Part print with two shaded views. Sizes in mm from the minimum x, y, z corner. Give positions to 0.01 mm unless a question says otherwise; leave off trailing zeros. Loops run counter-clockwise (first coordinate to the right, second up) from the corner with the lowest first, then second, coordinate; pieces in that order, holes last. Notation, with made-up numbers: (-34, -24.75) -> (3, -24.75) arc R16 cw to (3, -14.75) -> close; hole circle Ø9 at (36, 46). An arc over 180 degrees is marked (long way). One line per question, with ' | ' between items.
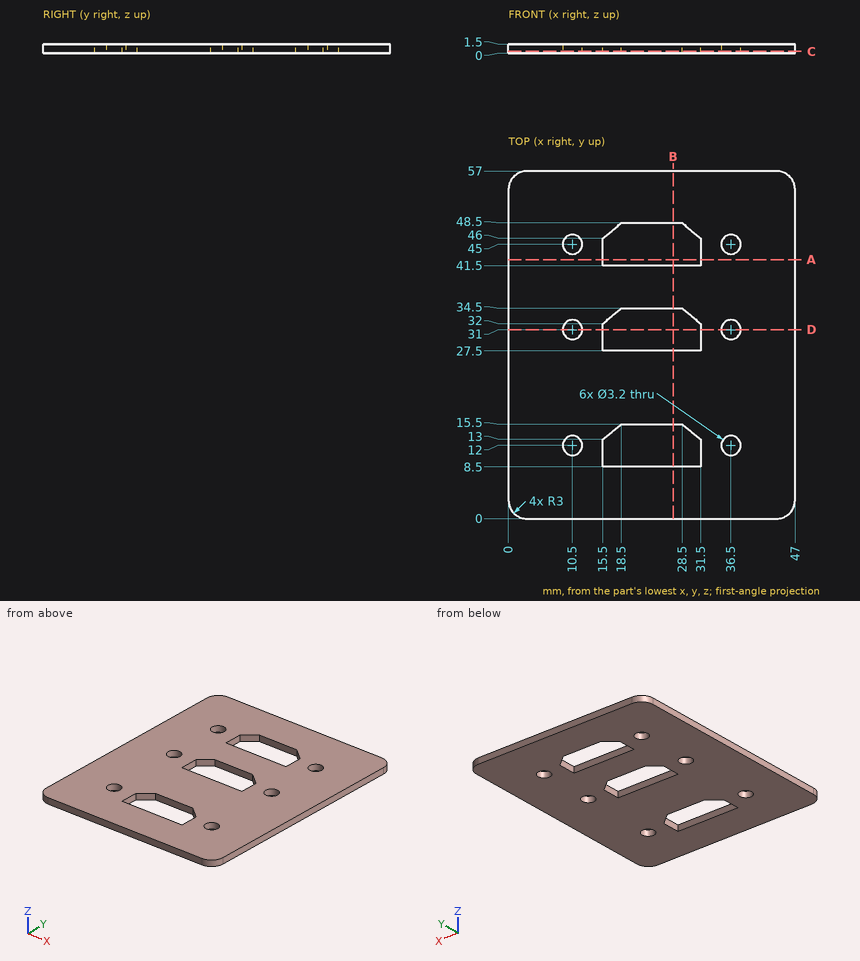
1) Saw through at A-A (y = 42.5). Give the cut face in (x, z), and give its area (3 significant figures).
Found:
outline: (0, 0) -> (15.5, 0) -> (15.5, 1.5) -> (0, 1.5) -> close; (31.5, 0) -> (47, 0) -> (47, 1.5) -> (31.5, 1.5) -> close | area: 46.5 mm2
2) Drill centre lines: line 1 (Y direction, x = 36.5, z = 0.75); line 2 (X direction, y = 9.5, z = 0.75); line 3 (X direction, y = 11, z = 0.65). Where is each one in solid material? Low to high.
Found:
line 1: 0 to 10.4, 13.6 to 29.4, 32.6 to 43.4, 46.6 to 57 | line 2: 0 to 15.5, 31.5 to 47 | line 3: 0 to 9.25, 11.75 to 15.5, 31.5 to 35.25, 37.75 to 47
3) Pin check, flat tip, straight feed: P1, Ø3, axis at x = 10.5, y = 12, coming from the +Z side. Stop position of the tip, or through.
Found:
P1: through
4) Saw through at D-D (y = 31). Give the cut face in (x, z), and give its area (3 significant figures).
Found:
outline: (0, 0) -> (8.9, 0) -> (8.9, 1.5) -> (0, 1.5) -> close; (12.1, 0) -> (15.5, 0) -> (15.5, 1.5) -> (12.1, 1.5) -> close; (31.5, 0) -> (34.9, 0) -> (34.9, 1.5) -> (31.5, 1.5) -> close; (38.1, 0) -> (47, 0) -> (47, 1.5) -> (38.1, 1.5) -> close | area: 36.9 mm2
5) Saw through at C-C (z = 0.3). State how many separate pieces and enclosed holes the cut face has, and give its area (3 significant figures).
Found:
separate pieces: 1 | enclosed holes: 9 | area: 2,310 mm2
6) Saw through at B-B (x = 27). Give the cut face in (y, z), and give its area (3 significant figures).
Found:
outline: (0, 0) -> (8.5, 0) -> (8.5, 1.5) -> (0, 1.5) -> close; (15.5, 0) -> (27.5, 0) -> (27.5, 1.5) -> (15.5, 1.5) -> close; (34.5, 0) -> (41.5, 0) -> (41.5, 1.5) -> (34.5, 1.5) -> close; (48.5, 0) -> (57, 0) -> (57, 1.5) -> (48.5, 1.5) -> close | area: 54.0 mm2
